from build123d import *

# Parameters (mm, degrees)
BOSS_EXTRUDE1_START = -18.956398
BOSS_EXTRUDE1_DEPTH = 6.000001


with BuildPart() as part:
    # Sketch1 → Boss-Extrude1 (new body)
    with BuildSketch(Plane.XY.offset(BOSS_EXTRUDE1_START)):
        with BuildLine():
            Line((144.558896816, -1449.426665995), (144.558896816, -1438.426665995))
            Line((144.558896816, -1438.426665995), (54.558896816, -1438.426665995))
            Line((54.558896816, -1438.426665995), (54.558896816, -1476.926665995))
            ThreePointArc((54.558896816, -1476.926665995), (55.619556988, -1477.366005823), (56.058896816, -1478.426665995))
            ThreePointArc((56.058896816, -1478.426665995), (54.558896816, -1479.926665995), (53.058896816, -1478.426665995))
            Line((53.058896816, -1478.426665995), (44.558896816, -1478.426665995))
            Line((44.558896816, -1478.426665995), (44.558896816, -1488.426665995))
            Line((44.558896816, -1488.426665995), (64.558896816, -1508.426665995))
            Line((64.558896816, -1508.426665995), (144.558896816, -1508.426665995))
            Line((144.558896816, -1508.426665995), (144.558896816, -1467.426665995))
            ThreePointArc((144.558896816, -1467.426665995), (135.558896816, -1458.426665995), (144.558896816, -1449.426665995))
        make_face()
        with BuildLine():
            Line((234.558896816, -1438.426665995), (144.558896816, -1438.426665995))
            Line((144.558896816, -1438.426665995), (144.558896816, -1449.426665995))
            ThreePointArc((144.558896816, -1449.426665995), (150.922857847, -1452.062704964), (153.558896816, -1458.426665995))
            ThreePointArc((153.558896816, -1458.426665995), (150.922857847, -1464.790627025), (144.558896816, -1467.426665995))
            Line((144.558896816, -1467.426665995), (144.558896816, -1508.426665995))
            Line((144.558896816, -1508.426665995), (224.558896816, -1508.426665995))
            Line((224.558896816, -1508.426665995), (244.558896816, -1488.426665995))
            Line((244.558896816, -1488.426665995), (244.558896816, -1478.426665995))
            Line((244.558896816, -1478.426665995), (236.058896816, -1478.426665995))
            ThreePointArc((236.058896816, -1478.426665995), (233.498236645, -1479.487326167), (234.558896816, -1476.926665995))
            Line((234.558896816, -1476.926665995), (234.558896816, -1438.426665995))
        make_face()
    extrude(amount=BOSS_EXTRUDE1_DEPTH)


solid = part.part
Geometry: final body of the model. Coordinates: model frame, mm. A direction names the side the tool comes from. Coordinates: 2 decimals unless noted, no trailing zeros. Order: outer loops, then holes, each group sorted by start corner. A loop starts at its lowest first (then second) coordinate and runs counter-clockwise, first axis right, second up.
1) Section A-A (z = -17). Return loops of the section in (x, y).
Result sheet:
outline: (44.56, -1488.43) - (64.56, -1508.43) - (224.56, -1508.43) - (244.56, -1488.43) - (244.56, -1478.43) - (236.06, -1478.43) arc R1.5 cw (long way) to (234.56, -1476.93) - (234.56, -1438.43) - (54.56, -1438.43) - (54.56, -1476.93) arc R1.5 cw (long way) to (53.06, -1478.43) - (44.56, -1478.43) - close; hole circle Ø18 at (144.56, -1458.43)
2) Ray query, probe 1 along X at (y, z) = (-1468, -14.75); probe 2 along Y at (x, z) = (139.5, -13.75); probe 3 along Y at (x, z) = (62, -14). Return the intervals inside material, ascending.
Result sheet:
probe 1: x = 54.56 to 234.56
probe 2: y = -1508.43 to -1465.87, -1450.98 to -1438.43
probe 3: y = -1505.87 to -1438.43
3) Section C-C (x = 149.5). Return loops of the section in (y, z), then the cut area to 3 significant figures.
Result sheet:
outline: (-1508.43, -18.96) - (-1465.95, -18.96) - (-1465.95, -12.96) - (-1508.43, -12.96) - close; (-1450.9, -18.96) - (-1438.43, -18.96) - (-1438.43, -12.96) - (-1450.9, -12.96) - close
area: 330 mm2
4) First-contact query: P1, Ø1, axis at y = -1466.5, z = -14, coming from the -X side. Flat tip, straight axial feed; report the tip coordinate or a pass-through.
Result sheet:
P1: stops at x = 54.56
5) Section D-D (y = -1494.5). Return loops of the section in (x, z), then the cut area to 3 significant figures.
Result sheet:
outline: (50.63, -18.96) - (238.49, -18.96) - (238.49, -12.96) - (50.63, -12.96) - close
area: 1,130 mm2
6) Set-up query: faces 4 (the flat face through (44.559, -1483, -16)), 5 (the flat face through (49, -1478.427, -16)), 6 (the flat face through (240, -1478.427, -16)). Return all of +Z, -Z, +X, -X, +Y, -Y with unobstructed straight access to the full face (end or side cutting, diameter ignored); none if empty.
Result sheet:
face 4: +Z, -Z, -X, +Y, -Y
face 5: +Z, -Z, -X, +Y
face 6: +Z, -Z, +X, +Y
7) Section B-B (y = -1451.5). Return loops of the section in (x, z).
Result sheet:
outline: (54.56, -18.96) - (138.81, -18.96) - (138.81, -12.96) - (54.56, -12.96) - close; (150.31, -18.96) - (234.56, -18.96) - (234.56, -12.96) - (150.31, -12.96) - close
8) Draft query along Z for faces 1 (the flat face through (143, -1473, -12.956)), 2 (the flat face through (244.559, -1483, -16)), 3 (the flat face through (143, -1473, -18.956)). Return one class per face: released by +Z, released by -Z, zero draft, split by the parting line, or undercut.
Result sheet:
face 1: released by +Z
face 2: zero draft
face 3: released by -Z
